```python
from build123d import *

# Parameters (mm, degrees)
EXTRUDE_1_DEPTH = 14
EXTRUDE_2_DEPTH = 71


with BuildPart() as part:
    # 草图1 → 凸台-拉伸1 (new body)
    with BuildSketch(Plane.XY):
        Polygon((71.4349048, -49.703584356), (71.4349048, -264.703584356), (11.4349048, -324.703584356), (-148.5650952, -234.703584356), (-148.5650952, 85.296415644), align=None)
    extrude(amount=EXTRUDE_1_DEPTH)

    # 草图2 → 凸台-拉伸2 (add)
    with BuildSketch(Plane.XY.offset(14)):
        Polygon((-134.5650952, 76.705506553), (-134.5650952, -242.578584356), (-148.5650952, -234.703584356), (-148.5650952, 85.296415644), align=None)
    extrude(amount=EXTRUDE_2_DEPTH)


solid = part.part
```
Here's how the part is built. I have some questions about the finished solid (model axes, mm). A direction names the side the tool comes from. Round coordinates to 2 decimals unless told otherwise and drop trailing zeros. Order: outer loops, then holes, each group sorted by start corner. A loop starts at its lowest first (then second) coordinate and runs counter-clockwise, first axis right, second up. Notation, with made-up numbers: M 57,-25 L 67,-25 A8 ccw 67,-19 Z; hole C 69.25,-8 d6. An arc over 180 degrees is marked long. Use CSV: the item, a comma, the result in double quotes.
1) I'm going to push flat-ended pins straight in: P1, Ø10, axis at x = -72, y = -161, coming from the +Z side; P2, Ø21.5, axis at y = -103.5, z = 38, coming from the +X side; P3, Ø5, axis at x = -10, z = 15, coming from the +Y side. Where does each tip first touch, or does it pass through?
Taken from the geometry:
P1,"z = 14"
P2,"x = -134.57"
P3,"y = 1.67"
2) I need wall thicknesses on line 1 along Z through (x, y) = (-29, -292); line 2 along X through (y, z) = (-38, 47.5); line 3 along Y through (x, z) = (59, 7.5). Which ranges of each line are inside material? Lowest first, please. Write a range as [from, to].
Taken from the geometry:
line 1,"[0, 14]"
line 2,"[-148.57, -134.57]"
line 3,"[-277.14, -42.07]"
3) I want a section at B-B (y = -195.5). List the corners of the cut face in (x, z) for me, then the cut area to 3 significant figures.
Taken from the geometry:
outline,"M -148.57,0 L 71.43,0 L 71.43,14 L -134.57,14 L -134.57,85 L -148.57,85 Z"
area,"4,070 mm^2"
4) I want a section at A-A (z = 6). List the corners of the cut face in (x, y) for me, then the cut area to 4 significant figures.
Taken from the geometry:
outline,"M -148.57,-234.7 L 11.43,-324.7 L 71.43,-264.7 L 71.43,-49.7 L -148.57,85.3 Z"
area,"66,350 mm^2"
5) I want a section at D-D (z = 52). List the corners of the cut face in (x, y) for me, then the cut area to 4 significant figures.
Taken from the geometry:
outline,"M -148.57,-234.7 L -134.57,-242.58 L -134.57,76.71 L -148.57,85.3 Z"
area,"4,475 mm^2"
6) On a 3-axis mill with a long thin cutter (end or side, diameter ignored), from which of +Z, -Z, +X, -X, +Y, -Y can I reach the whole of each face in a straight line? I mean faces 1 (the flat face through (-134.565, -81, 49)), 2 (the flat face through (-37, -117, 0)). Say none if no direction works.
Taken from the geometry:
face 1,"+Z, +X, +Y, -Y"
face 2,"-Z, +X, -X, +Y, -Y"
7) If we mould it in two halves opening along X, with no side actions, what happens to faces 3 (the flat face through (-30, -121, 14)), 4 (the flat face through (71.435, -156, 7)), 5 (the flat face through (-91.895, -266.58, 10.82))? For each: pulls with the +X half, pulls with the -X half, needs draft (parallel to the pull), parting line crosses it, or undercut.
Taken from the geometry:
face 3,"needs draft"
face 4,"pulls with the +X half"
face 5,"pulls with the -X half"
8) I want a section at C-C (x = -116). List the corners of the cut face in (y, z) for me, then the cut area to 3 significant figures.
Taken from the geometry:
outline,"M -253.02,0 L 65.31,0 L 65.31,14 L -253.02,14 Z"
area,"4,460 mm^2"
